The model under review builds one solid part; all positions refer to its coordinate system, in mm. Face numbers are marked on the shaded views. Coordinates: 2 decimals unless noted, no trailing zeros. Order: outer loops, then holes, each group sorted by start corner. A loop starts at its lowest first (then second) coordinate and runs counter-clockwise, first axis right, second up. Notation, with made-up numbers: (-16, 82.25) -> (3, 82.25) arc R32 cw to (3, 108.25) -> close; hole circle Ø3 at (-28, -8.75). An arc over 180 degrees is marked (long way). Put each result on its own line as item: value.
from build123d import *

# Parameters (mm, degrees)
SKETCH1_R                                      = 16.5
BOSS_EXTRUDE1_DEPTH                            = 3
SKETCH2_R                                      = 3
BOSS_EXTRUDE2_DEPTH                            = 12
SKETCH3_R                                      = 6
BOSS_EXTRUDE3_DEPTH                            = 1
CUT_EXTRUDE1_START                             = -11
CUT_EXTRUDE1_DEPTH                             = 11
SKETCH5_R                                      = 2
CUT_EXTRUDE2_DEPTH                             = 27.239283527
CIRPATTERN1_COUNT                              = 4
CSK_FOR_M4_FLAT_HEAD_MACHINE_SCREW1_AT_2_COUNT = 2
CSK_FOR_M4_FLAT_HEAD_MACHINE_SCREW1_AT_2_PITCH = 16.263455967
CSK_FOR_M4_FLAT_HEAD_MACHINE_SCREW1_AT_3_COUNT = 2
CSK_FOR_M4_FLAT_HEAD_MACHINE_SCREW1_AT_3_PITCH = 23
CSK_FOR_M4_FLAT_HEAD_MACHINE_SCREW1_AT_4_COUNT = 2
CSK_FOR_M4_FLAT_HEAD_MACHINE_SCREW1_AT_4_PITCH = 16.263455967
CUT_EXTRUDE3_START                             = -1
SKETCH9_R                                      = 6
CUT_EXTRUDE3_DEPTH                             = 1
SKETCH10_W                                     = 0.3
SKETCH10_H                                     = 0.4


with BuildPart() as part:
    # Sketch1 → Boss-Extrude1 (new body)
    with BuildSketch(Plane.XY):
        Circle(SKETCH1_R)
    extrude(amount=BOSS_EXTRUDE1_DEPTH)

    # Sketch2 → Boss-Extrude2 (add)
    with BuildSketch(Plane.XY.offset(3)):
        Circle(SKETCH2_R)
    extrude(amount=BOSS_EXTRUDE2_DEPTH)

    # Sketch3 → Boss-Extrude3 (add)
    with BuildSketch(Plane.XY.offset(3)):
        Circle(SKETCH3_R)
    extrude(amount=BOSS_EXTRUDE3_DEPTH)

    # Sketch4 → Cut-Extrude1 (cut)
    with BuildSketch(Plane.XY.offset(15).offset(CUT_EXTRUDE1_START)):
        with BuildLine():
            Line((-2.5, -1.658312395), (-2.5, 1.658312395))
            ThreePointArc((-2.5, 1.658312395), (-3, 0), (-2.5, -1.658312395))
        make_face()
    extrude(amount=CUT_EXTRUDE1_DEPTH, mode=Mode.SUBTRACT)

    # Sketch5 → Cut-Extrude2 (cut, through all)
    with BuildSketch(Plane.XY.offset(3)):
        with Locations((0, 11.5)):
            Circle(SKETCH5_R)
    cut_extrude2 = extrude(amount=-CUT_EXTRUDE2_DEPTH, mode=Mode.SUBTRACT)

    # CirPattern1: Cut-Extrude2 ×4 about axis
    cirpattern1_axis = Axis((0, 0, 0), (0, 0, 1))
    for i in range(1, CIRPATTERN1_COUNT):
        add(cut_extrude2.rotate(cirpattern1_axis, i * 360 / CIRPATTERN1_COUNT), mode=Mode.SUBTRACT)

    # Sketch8 → CSK for M4 Flat Head Machine Screw1 (revolve, cut)
    with BuildSketch(Plane(origin=(-11.5, 0, 3), x_dir=(0, -1, 0), z_dir=(1, 0, 0))):
        Polygon((0, 0), (0, 3), (2.25, 3), (2.25, 2.45), (4.7, 0), align=None)
    csk_for_m4_flat_head_machine_screw1 = revolve(axis=Axis((-11.5, 0, 9.35), (0, 0, -1)), mode=Mode.SUBTRACT)

    # CSK for M4 Flat Head Machine Screw1 at 2: CSK for M4 Flat Head Machine Screw1 ×2
    with Locations(*[Vector(0.7071067811865462, 0.7071067811865488, 0) * (i * CSK_FOR_M4_FLAT_HEAD_MACHINE_SCREW1_AT_2_PITCH) for i in range(1, CSK_FOR_M4_FLAT_HEAD_MACHINE_SCREW1_AT_2_COUNT)]):
        add(csk_for_m4_flat_head_machine_screw1, mode=Mode.SUBTRACT)

    # CSK for M4 Flat Head Machine Screw1 at 3: CSK for M4 Flat Head Machine Screw1 ×2
    with Locations(*[(i * CSK_FOR_M4_FLAT_HEAD_MACHINE_SCREW1_AT_3_PITCH, 0, 0) for i in range(1, CSK_FOR_M4_FLAT_HEAD_MACHINE_SCREW1_AT_3_COUNT)]):
        add(csk_for_m4_flat_head_machine_screw1, mode=Mode.SUBTRACT)

    # CSK for M4 Flat Head Machine Screw1 at 4: CSK for M4 Flat Head Machine Screw1 ×2
    with Locations(*[Vector(0.7071067811865488, -0.7071067811865462, 0) * (i * CSK_FOR_M4_FLAT_HEAD_MACHINE_SCREW1_AT_4_PITCH) for i in range(1, CSK_FOR_M4_FLAT_HEAD_MACHINE_SCREW1_AT_4_COUNT)]):
        add(csk_for_m4_flat_head_machine_screw1, mode=Mode.SUBTRACT)

    # Sketch9 → Cut-Extrude3 (cut)
    with BuildSketch(Plane.XY.offset(4).offset(CUT_EXTRUDE3_START)):
        Circle(SKETCH9_R)
        with BuildLine():
            Line((-2.5, -1.658312395), (-2.5, 1.658312395))
            ThreePointArc((-2.5, 1.658312395), (3, 0), (-2.5, -1.658312395))
        make_face(mode=Mode.SUBTRACT)
    extrude(amount=CUT_EXTRUDE3_DEPTH, mode=Mode.SUBTRACT)

    # Sketch10 → Cut-Revolve1 (revolve, cut)
    with BuildSketch(Plane(origin=(0, 0, 0), x_dir=(1, 0, 0), z_dir=(0, 1, 0))):
        with Locations((3, -11.2)):
            Rectangle(SKETCH10_W, SKETCH10_H)
    revolve(axis=Axis((0, 0, 0), (0, 0, 1)), mode=Mode.SUBTRACT)


solid = part.part
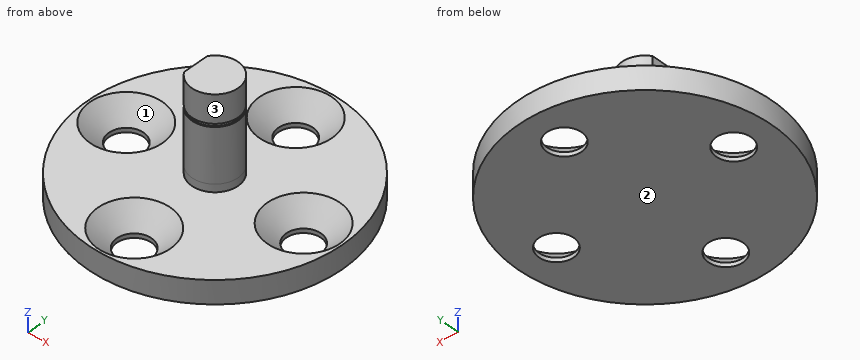
Item 1: For line 1 (Y direction, x = 0, z = 0.3); line 2 (Y direction, x = 1.5, z = 1.25); line 3 (Z direction, x = -5, y = -8), list the stretches that pass through material, from the lowest coordinate up. Write a range as from..to.
Answers below:
line 1: -16.5..-13.75, -9.25..9.25, 13.75..16.5
line 2: -16.43..-14.04, -8.96..8.96, 14.04..16.43
line 3: 0..3
Item 2: Consider section A-A on y = 0. Write out the cut boundary in (x, z).
Answers below:
outline: (-16.5, 0) -> (-13.75, 0) -> (-13.75, 0.55) -> (-16.2, 3) -> (-16.5, 3) -> close; (-9.25, 0) -> (9.25, 0) -> (9.25, 0.55) -> (6.8, 3) -> (3, 3) -> (3, 11) -> (2.85, 11) -> (2.85, 11.4) -> (3, 11.4) -> (3, 15) -> (-2.5, 15) -> (-2.5, 3) -> (-6.8, 3) -> (-9.25, 0.55) -> close; (13.75, 0) -> (16.5, 0) -> (16.5, 3) -> (16.2, 3) -> (13.75, 0.55) -> close
Item 3: For pin 1 Ø2.5 at (y, z) = (0.5, 11.5) entering from -X; pin 2 Ø5 at (x, y) = (0, 11.5) entering from +Z; pin 3 Ø3 at (y, z) = (-7, 3.5) entering from +X, all flat-tipped, find the tip position at first contact; note any pin that passes through.
Answers below:
pin 1: x = -2.5
pin 2: z = 0.8
pin 3: x = 15.53
Item 4: Mouldability with a two-part tool opening along Y and no side actions: class the marked faces 1, 2 and 3 as +Y half, -Y half, draft (parallel to the pull), parting line (faces both ways), or undercut.
Answers below:
face 1: undercut
face 2: draft
face 3: parting line
Item 5: Consider section B-B on x = 0. Write out the cut boundary in (y, z).
Answers below:
outline: (-16.5, 0) -> (-13.75, 0) -> (-13.75, 0.55) -> (-16.2, 3) -> (-16.5, 3) -> close; (-9.25, 0) -> (9.25, 0) -> (9.25, 0.55) -> (6.8, 3) -> (3, 3) -> (3, 11) -> (2.85, 11) -> (2.85, 11.4) -> (3, 11.4) -> (3, 15) -> (-3, 15) -> (-3, 11.4) -> (-2.85, 11.4) -> (-2.85, 11) -> (-3, 11) -> (-3, 3) -> (-6.8, 3) -> (-9.25, 0.55) -> close; (13.75, 0) -> (16.5, 0) -> (16.5, 3) -> (16.2, 3) -> (13.75, 0.55) -> close
Item 6: Consider section C-C on x = 11.5. Write out the cut boundary in (y, z).
Answers below:
outline: (-11.83, 0) -> (-2.25, 0) -> (-2.25, 0.55) -> (-4.7, 3) -> (-11.83, 3) -> close; (2.25, 0) -> (11.83, 0) -> (11.83, 3) -> (4.7, 3) -> (2.25, 0.55) -> close
